Design review of the part built by this model. Coordinates are the model's own, in mm. A direction names the side the tool comes from. Coordinates: 2 decimals unless noted, no trailing zeros. Write each loop counter-clockwise with the first axis right and the second up, starting at its lowest first coordinate (ties: lowest second). Pieces come first, ordered by that corner, then holes. Notation, with made-up numbers: (0.25, 11.25) - (31.25, 11.25) arc R18 ccw to (31.25, 32.25) - close; hole circle Ø10 at (60, -36.75). An arc over 180 degrees is marked (long way). One line per item, written item: value.
from build123d import *

# Parameters (mm, degrees)
F0_W      = 20
F0_H      = 20
F1_DEPTH  = 0.85
F1_FACE_W = 20
F1_FACE_H = 20
F2_DEPTH  = 1
F3_D      = 5


with BuildPart() as f1:
    # F0 (on Top) → F1 (new body)
    with BuildSketch(Plane.XY):
        Polygon((-125, 52), (-177, 52), (-177, -22), (-125, -22), (-125, 0), (-80, 0), (-80, -22), (22, -22), (22, 52), (-80, 52), (-80, 30), (-125, 30), align=None)
        with Locations((-165, -10)):
            Rectangle(F0_W, F0_H, mode=Mode.SUBTRACT)
        with Locations((-140, -10)):
            Rectangle(F0_W, F0_H, mode=Mode.SUBTRACT)
        with Locations((-65, -10)):
            Rectangle(F0_W, F0_H, mode=Mode.SUBTRACT)
        with Locations((-40, -10)):
            Rectangle(F0_W, F0_H, mode=Mode.SUBTRACT)
        with Locations((-15, -10)):
            Rectangle(F0_W, F0_H, mode=Mode.SUBTRACT)
        with Locations((10, -10)):
            Rectangle(F0_W, F0_H, mode=Mode.SUBTRACT)
        with Locations((-165, 15)):
            Rectangle(F0_W, F0_H, mode=Mode.SUBTRACT)
        with Locations((-140, 15)):
            Rectangle(F0_W, F0_H, mode=Mode.SUBTRACT)
        with Locations((-115, 15)):
            Rectangle(F0_W, F0_H, mode=Mode.SUBTRACT)
        with Locations((-90, 15)):
            Rectangle(F0_W, F0_H, mode=Mode.SUBTRACT)
        with Locations((-165, 40)):
            Rectangle(F0_W, F0_H, mode=Mode.SUBTRACT)
        with Locations((-140, 40)):
            Rectangle(F0_W, F0_H, mode=Mode.SUBTRACT)
        with Locations((-65, 15)):
            Rectangle(F0_W, F0_H, mode=Mode.SUBTRACT)
        with Locations((-40, 15)):
            Rectangle(F0_W, F0_H, mode=Mode.SUBTRACT)
        with Locations((-15, 15)):
            Rectangle(F0_W, F0_H, mode=Mode.SUBTRACT)
        with Locations((10, 15)):
            Rectangle(F0_W, F0_H, mode=Mode.SUBTRACT)
        with Locations((-65, 40)):
            Rectangle(F0_W, F0_H, mode=Mode.SUBTRACT)
        with Locations((-40, 40)):
            Rectangle(F0_W, F0_H, mode=Mode.SUBTRACT)
        with Locations((-15, 40)):
            Rectangle(F0_W, F0_H, mode=Mode.SUBTRACT)
        with Locations((10, 40)):
            Rectangle(F0_W, F0_H, mode=Mode.SUBTRACT)
    extrude(amount=F1_DEPTH)

    # F0 (on Top) + F1_face (on face) → F2 (join)
    with BuildSketch(Plane.XY):
        Polygon((-125, 52), (-177, 52), (-177, -22), (-125, -22), (-125, 0), (-80, 0), (-80, -22), (22, -22), (22, 52), (-80, 52), (-80, 30), (-125, 30), align=None)
        with Locations((-165, -10)):
            Rectangle(F0_W, F0_H, mode=Mode.SUBTRACT)
        with Locations((-140, -10)):
            Rectangle(F0_W, F0_H, mode=Mode.SUBTRACT)
        with Locations((-65, -10)):
            Rectangle(F0_W, F0_H, mode=Mode.SUBTRACT)
        with Locations((-40, -10)):
            Rectangle(F0_W, F0_H, mode=Mode.SUBTRACT)
        with Locations((-15, -10)):
            Rectangle(F0_W, F0_H, mode=Mode.SUBTRACT)
        with Locations((10, -10)):
            Rectangle(F0_W, F0_H, mode=Mode.SUBTRACT)
        with Locations((-165, 15)):
            Rectangle(F0_W, F0_H, mode=Mode.SUBTRACT)
        with Locations((-140, 15)):
            Rectangle(F0_W, F0_H, mode=Mode.SUBTRACT)
        with Locations((-115, 15)):
            Rectangle(F0_W, F0_H, mode=Mode.SUBTRACT)
        with Locations((-90, 15)):
            Rectangle(F0_W, F0_H, mode=Mode.SUBTRACT)
        with Locations((-165, 40)):
            Rectangle(F0_W, F0_H, mode=Mode.SUBTRACT)
        with Locations((-140, 40)):
            Rectangle(F0_W, F0_H, mode=Mode.SUBTRACT)
        with Locations((-65, 15)):
            Rectangle(F0_W, F0_H, mode=Mode.SUBTRACT)
        with Locations((-40, 15)):
            Rectangle(F0_W, F0_H, mode=Mode.SUBTRACT)
        with Locations((-15, 15)):
            Rectangle(F0_W, F0_H, mode=Mode.SUBTRACT)
        with Locations((10, 15)):
            Rectangle(F0_W, F0_H, mode=Mode.SUBTRACT)
        with Locations((-65, 40)):
            Rectangle(F0_W, F0_H, mode=Mode.SUBTRACT)
        with Locations((-40, 40)):
            Rectangle(F0_W, F0_H, mode=Mode.SUBTRACT)
        with Locations((-15, 40)):
            Rectangle(F0_W, F0_H, mode=Mode.SUBTRACT)
        with Locations((10, 40)):
            Rectangle(F0_W, F0_H, mode=Mode.SUBTRACT)
        with Locations((-140, 15)):
            Rectangle(F0_W, F0_H)
        with Locations((-165, 15)):
            Rectangle(F0_W, F0_H)
        with Locations((-165, 40)):
            Rectangle(F0_W, F0_H)
        with Locations((-140, 40)):
            Rectangle(F0_W, F0_H)
        with Locations((-115, 15)):
            Rectangle(F0_W, F0_H)
        with Locations((-140, -10)):
            Rectangle(F0_W, F0_H)
        with Locations((-165, -10)):
            Rectangle(F0_W, F0_H)
        with Locations((-90, 15)):
            Rectangle(F0_W, F0_H)
        with Locations((-65, 40)):
            Rectangle(F0_W, F0_H)
        with Locations((-65, 15)):
            Rectangle(F0_W, F0_H)
        with Locations((-40, 15)):
            Rectangle(F0_W, F0_H)
        with Locations((-65, -10)):
            Rectangle(F0_W, F0_H)
        with Locations((-40, -10)):
            Rectangle(F0_W, F0_H)
        with Locations((-40, 40)):
            Rectangle(F0_W, F0_H)
        with Locations((-15, 40)):
            Rectangle(F0_W, F0_H)
        with Locations((-15, 15)):
            Rectangle(F0_W, F0_H)
        with Locations((-15, -10)):
            Rectangle(F0_W, F0_H)
        with Locations((10, -10)):
            Rectangle(F0_W, F0_H)
        with Locations((10, 15)):
            Rectangle(F0_W, F0_H)
        with Locations((10, 40)):
            Rectangle(F0_W, F0_H)
    with BuildSketch(Plane(origin=(-75.49831437, 15, 0.85), x_dir=(1, 0, 0), z_dir=(0, 0, 1))):
        Polygon((-49.50168563, 37), (-101.50168563, 37), (-101.50168563, -37), (-49.50168563, -37), (-49.50168563, -15), (-4.50168563, -15), (-4.50168563, -37), (97.49831437, -37), (97.49831437, 37), (-4.50168563, 37), (-4.50168563, 15), (-49.50168563, 15), align=None)
        with Locations((-89.50168563, -25)):
            Rectangle(F1_FACE_W, F1_FACE_H, mode=Mode.SUBTRACT)
        with Locations((-64.50168563, -25)):
            Rectangle(F1_FACE_W, F1_FACE_H, mode=Mode.SUBTRACT)
        with Locations((10.49831437, -25)):
            Rectangle(F1_FACE_W, F1_FACE_H, mode=Mode.SUBTRACT)
        with Locations((35.49831437, -25)):
            Rectangle(F1_FACE_W, F1_FACE_H, mode=Mode.SUBTRACT)
        with Locations((60.49831437, -25)):
            Rectangle(F1_FACE_W, F1_FACE_H, mode=Mode.SUBTRACT)
        with Locations((85.49831437, -25)):
            Rectangle(F1_FACE_W, F1_FACE_H, mode=Mode.SUBTRACT)
        with Locations((-89.50168563, 0)):
            Rectangle(F1_FACE_W, F1_FACE_H, mode=Mode.SUBTRACT)
        with Locations((-64.50168563, 0)):
            Rectangle(F1_FACE_W, F1_FACE_H, mode=Mode.SUBTRACT)
        with Locations((-39.50168563, 0)):
            Rectangle(F1_FACE_W, F1_FACE_H, mode=Mode.SUBTRACT)
        with Locations((-14.50168563, 0)):
            Rectangle(F1_FACE_W, F1_FACE_H, mode=Mode.SUBTRACT)
        with Locations((-89.50168563, 25)):
            Rectangle(F1_FACE_W, F1_FACE_H, mode=Mode.SUBTRACT)
        with Locations((-64.50168563, 25)):
            Rectangle(F1_FACE_W, F1_FACE_H, mode=Mode.SUBTRACT)
        with Locations((10.49831437, 0)):
            Rectangle(F1_FACE_W, F1_FACE_H, mode=Mode.SUBTRACT)
        with Locations((35.49831437, 0)):
            Rectangle(F1_FACE_W, F1_FACE_H, mode=Mode.SUBTRACT)
        with Locations((60.49831437, 0)):
            Rectangle(F1_FACE_W, F1_FACE_H, mode=Mode.SUBTRACT)
        with Locations((85.49831437, 0)):
            Rectangle(F1_FACE_W, F1_FACE_H, mode=Mode.SUBTRACT)
        with Locations((10.49831437, 25)):
            Rectangle(F1_FACE_W, F1_FACE_H, mode=Mode.SUBTRACT)
        with Locations((35.49831437, 25)):
            Rectangle(F1_FACE_W, F1_FACE_H, mode=Mode.SUBTRACT)
        with Locations((60.49831437, 25)):
            Rectangle(F1_FACE_W, F1_FACE_H, mode=Mode.SUBTRACT)
        with Locations((85.49831437, 25)):
            Rectangle(F1_FACE_W, F1_FACE_H, mode=Mode.SUBTRACT)
    extrude(amount=-F2_DEPTH)

    # F3 (through all)
    with Locations(Plane.XY):
        with Locations((-140, 40), (-140, -10), (-65, 15), (10, -10), (10, 40)):
            Hole(F3_D / 2)


solid = f1.part
1. Insertion check: pin 1 Ø5 at (x, y) = (-108, 13.5) entering from +Z. The pin has a flat end and moves straight along its axis. Give the tip position at first contact, or say it passes through.
Answer block:
pin 1: stops at z = 0
2. Consider section C-C, the plane y = -10. Give the number of separate pieces and of enclosed holes in the cut face, then the cut area to 3 significant figures.
Answer block:
separate pieces: 4
enclosed holes: 0
area: 173 mm^2
3. Consider section D-D, the plane x = -109.5. Write out the cut boundary in (y, z), then the cut area to 3 significant figures.
Answer block:
outline: (0, -1) - (30, -1) - (30, 0.85) - (25, 0.85) - (25, 0) - (5, 0) - (5, 0.85) - (0, 0.85) - close
area: 38.5 mm^2
4. Mouldability with a two-part tool opening along Y and no side actions: class faces 1 (the face through (-63, 13, 0)), 2 (the face through (12, 42, 0)), 3 (the face through (-79, 16, -1)) as released by +Y, released by -Y, zero draft, split by the parting line, or undercut.
Answer block:
face 1: undercut
face 2: undercut
face 3: zero draft
5. Consider section B-B, the plane x = -47. Write out the cut boundary in (y, z), then the cut area to 3 significant figures.
Answer block:
outline: (-22, -1) - (52, -1) - (52, 0.85) - (50, 0.85) - (50, 0) - (30, 0) - (30, 0.85) - (25, 0.85) - (25, 0) - (5, 0) - (5, 0.85) - (0, 0.85) - (0, 0) - (-20, 0) - (-20, 0.85) - (-22, 0.85) - close
area: 85.9 mm^2
6. Wall thickness on line 1 along Y through (x, z) = (-140, -0.35); line 2 along Y through (x, z) = (-65, -0.7); line 3 along X through (y, z) = (34, -0.7): over which ranges is each line inside the solid? List them lowest first.
Answer block:
line 1: y = -22 to -12.5, -7.5 to 37.5, 42.5 to 52
line 2: y = -22 to 12.5, 17.5 to 52
line 3: x = -177 to -125, -80 to 22
7. For faces 4 (the face through (-40, -10, 0)), 5 (the face through (-78, 18, 0.85)), list the 3-axis set-ups (+Z, -Z, +X, -X, +Y, -Y) from which the entire face can be reached by the end or side of a thin tool; tool diameter is ignored.
Answer block:
face 4: +Z
face 5: +Z, +X, -X, +Y, -Y
8. Consider section A-A, the plane x = -140. Write out the cut boundary in (y, z).
Answer block:
outline: (-22, -1) - (-12.5, -1) - (-12.5, 0) - (-20, 0) - (-20, 0.85) - (-22, 0.85) - close; (-7.5, -1) - (37.5, -1) - (37.5, 0) - (30, 0) - (30, 0.85) - (25, 0.85) - (25, 0) - (5, 0) - (5, 0.85) - (0, 0.85) - (0, 0) - (-7.5, 0) - close; (42.5, -1) - (52, -1) - (52, 0.85) - (50, 0.85) - (50, 0) - (42.5, 0) - close
